Geometry: final body of the model. Coordinates: model frame, mm. A direction names the side the tool comes from. Coordinates: 2 decimals unless noted, no trailing zeros. Order: outer loops, then holes, each group sorted by start corner. A loop starts at its lowest first (then second) coordinate and runs counter-clockwise, first axis right, second up. Notation, with made-up numbers: M 88.5,71.5 L 139.5,71.5 A18 ccw 139.5,100.5 Z; hole C 68.25,-11 d6. An arc over 180 degrees is marked long. Use CSV: the item, a comma, the result in double quotes. Start each with the question number.
1. Section query A-A on x = 0. Return the cut outline in (y, z).
2. Set-up query: faces 5 (the cylindrical face through (10, 0, 7)), 6 (the flat face through (-17.25, -8.973, 2.465)). Return all of +Z, -Z, +X, -X, +Y, -Y with unobstructed straight access to the full face (end or side cutting, diameter ignored); none if empty.
3. Pull-direction query (Y, two-part tool) for faces 1 (the cylindrical face through (-26.343, -0.192, 2.465)), 2 (the cylindrical face through (-1.962, -8.837, 12.465)), 3 (the flat face through (2, -9, 10)), 4 (the cylindrical face through (-7.493, 0.33, 2.465)); classes: pulls with the +Y half, pulls with the -Y half, needs draft (parallel to the pull), parting line crosses it, or undercut.
4. First-contact query: P1, Ø9, axis at x = -22.85, y = -0.35, coming from the +Z side; P2, Ø6, axis at y = -5.5, z = 9, coming from the -X side; P3, Ø12, axis at x = 0, y = 0, coming from the +Z side. Flat tips, straight axial feed; report the tip coordinate or a pass-through.
5. Section query C-C on z = 2. Return the cut outline in (x, y), and give its area (3 significant figures).
6. Section query B-B on z = 8. Return the cut outline in (x, y).
7. Section query D-D on x = -25.5. Return the cut outline in (y, z).
8. Material intervals for line 1 (Y direction, x = 0, z = 3.6); line 2 (Y direction, x = 0, z = 7.45); line 3 (Z direction, x = -8, y = -8), sorted ascending.
from build123d import *

# Parameters (mm, degrees)
SKETCH2_R           = 7.5
SKETCH2_R_2         = 3.5
BOSS_EXTRUDE1_DEPTH = 5
SKETCH3_R           = 10
SKETCH3_R_2         = 6.052399113
BOSS_EXTRUDE2_DEPTH = 5
SKETCH5_R           = 9.052399113
SKETCH5_R_2         = 7.5
BOSS_EXTRUDE3_DEPTH = 5


with BuildPart() as part:
    # Sketch2 → Boss-Extrude1 (new body)
    with BuildSketch(Plane.XY):
        with BuildLine():
            Line((-32.094512491, 4.68250523), (-3.101754703, 12.109051068))
            ThreePointArc((-3.101754703, 12.109051068), (-0.215678408, 12.498139174), (2.682104326, 12.208862207))
            Line((2.682104326, 12.208862207), (32.368196231, 5.687272056))
            ThreePointArc((32.368196231, 5.687272056), (32.932912283, 5.337233509), (33.153627885, 4.710563079))
            Line((33.153627885, 4.710563079), (33.153627885, -3.707266727))
            ThreePointArc((33.153627885, -3.707266727), (32.942891731, -4.321320943), (32.399502723, -4.676568312))
            Line((32.399502723, -4.676568312), (2.938551053, -12.149687967))
            ThreePointArc((2.938551053, -12.149687967), (0.047582142, -12.499909437), (-2.845969256, -12.171707316))
            Line((-2.845969256, -12.171707316), (-32.063143376, -5.684001735))
            ThreePointArc((-32.063143376, -5.684001735), (-32.626362904, -5.333570306), (-32.846372115, -4.707779311))
            Line((-32.846372115, -4.707779311), (-32.846372115, 3.713781144))
            ThreePointArc((-32.846372115, 3.713781144), (-32.636353246, 4.326912298), (-32.094512491, 4.68250523))
        make_face()
        Circle(SKETCH2_R, mode=Mode.SUBTRACT)
        with Locations((-22.846372115, -0.345688892)):
            Circle(SKETCH2_R_2, mode=Mode.SUBTRACT)
        with Locations((23.153627885, 0.350337985)):
            Circle(SKETCH2_R_2, mode=Mode.SUBTRACT)
    extrude(amount=BOSS_EXTRUDE1_DEPTH)

    # Sketch3 → Boss-Extrude2 (add)
    with BuildSketch(Plane.XY.offset(5)):
        with Locations(Location((0, 0, 0), (0, 0, 180))):
            Circle(SKETCH3_R)
        Circle(SKETCH3_R_2, mode=Mode.SUBTRACT)
    extrude(amount=BOSS_EXTRUDE2_DEPTH)

    # Sketch5 → Boss-Extrude3 (add)
    with BuildSketch(Plane.XY.offset(10)):
        Circle(SKETCH5_R)
        Circle(SKETCH5_R_2, mode=Mode.SUBTRACT)
    extrude(amount=BOSS_EXTRUDE3_DEPTH)


solid = part.part
Results list:
1,outline,"M -12.5,0 L -7.5,0 L -7.5,5 L -6.05,5 L -6.05,10 L -7.5,10 L -7.5,15 L -9.05,15 L -9.05,10 L -10,10 L -10,5 L -12.5,5 Z; M 6.05,5 L 7.5,5 L 7.5,0 L 12.5,0 L 12.5,5 L 10,5 L 10,10 L 9.05,10 L 9.05,15 L 7.5,15 L 7.5,10 L 6.05,10 Z"
2,face 5,"+Z"
2,face 6,"+Z, -Z, -X, -Y"
3,face 1,"undercut"
3,face 2,"parting line crosses it"
3,face 3,"needs draft"
3,face 4,"undercut"
4,P1,"stops at z = 5"
4,P2,"stops at x = -9.68"
4,P3,"passes through"
5,outline,"M -32.85,-4.71 A1 ccw -32.06,-5.68 L -2.85,-12.17 A12.5 ccw 2.94,-12.15 L 32.4,-4.68 A1 ccw 33.15,-3.71 L 33.15,4.71 A1 ccw 32.37,5.69 L 2.68,12.21 A12.5 ccw -3.1,12.11 L -32.09,4.68 A1 ccw -32.85,3.71 Z; hole C -22.85,-0.35 d7; hole C 0,0 d15; hole C 23.15,0.35 d7"
5,area,"923 mm²"
6,outline,"C 0,0 d20; hole C 0,0 d12.1"
7,outline,"M -7.14,0 L -2.63,0 L -2.63,5 L -7.14,5 Z; M 1.94,0 L 6.37,0 L 6.37,5 L 1.94,5 Z"
8,line 1,"y = -12.5 to -7.5, 7.5 to 12.5"
8,line 2,"y = -10 to -6.05, 6.05 to 10"
8,line 3,"z = 0 to 5"
